Work out the finished part from the listing and answer in its coordinate system (mm). A direction names the side the tool comes from. Give positions to 0.01 mm unless a question says otherwise; leave off trailing zeros. Loops run counter-clockwise (first coordinate to the right, second up) from the corner with the lowest first, then second, coordinate; pieces in that order, holes last. Notation, with made-up numbers: (39.5, 39.25) - (50.5, 39.25) arc R9 ccw to (50.5, 53.25) - close; hole circle Ø7 at (-24, -35.75). An arc over 180 degrees is marked (long way). One line per question, with ' | ' between items. Start each with the question number.
1. Which of the six approach directions +Z, -Z, +X, -X, +Y, -Y give full straight-line access (tool end or side, diameter ignored) to faces 1 (the face through (-69, -3.44, 3)), 2 (the face through (-65.085, -17, 3)), 3 (the face through (-63, -9, 3))?
2. Section B-B (x = -4) is taken. Determine the outline of the cut face in (y, z), plus the area to 3 significant figures.
3. Section C-C (y = 10) is taken. Determine the outline of the cut face in (x, z) (3 decimals), plus the area to 3 significant figures.
4. Each of these flat-tipped pins is pushed along its axis until it touches: pin 1 (2 mm diameter, centred on y = -1.5, z = 4, fed in from -X); pin 2 (1 mm diameter, centred on x = -46.5, z = 3, fed in from +Y). Where does it stop, or does it pass through?
5. Section D-D (z = 3.75) is taken. Give the number of separate pieces and of enclosed holes in the cut face, plus the area to 3 significant figures.
6. Section A-A (y = -10) is taken. Determine the outline of the cut face in (x, z) (3 decimals), plus the area to 3 significant figures.
7. Find the intervals of material crossed by line 1 (Y direction, x = 21, z = 3.75) (3 decimals); line 2 (Y direction, x = -21, z = 3.5) (3 decimals); line 3 (Y direction, x = -2.5, z = 5.25), in increasing order.
8. For a pull along Y with two mould halves and no side action, classify faces 4 (the face through (-45.2, 40.1, 3.3)), 5 (the face through (-22.31, 11.2, 3.25)), 6 (the face through (-50.3, 20, 3)) as released by +Y, released by -Y, zero draft, split by the parting line, or undercut.
from build123d import *

# Parameters (mm, degrees)
MODEL_R             = 1.775
MODEL_W             = 28.5
MODEL_H             = 6.88
BOSS_EXTRUDE1_DEPTH = 6.6


with BuildPart() as part:
    # Model → Boss-Extrude1 (new body)
    with BuildSketch(Plane.XY):
        with BuildLine():
            Line((-40.3, 45), (-50.3, 35))
            Line((-50.3, 35), (-50.3, 5.44))
            ThreePointArc((-50.3, 5.44), (-49.714213562, 4.025786438), (-48.3, 3.44))
            Line((-48.3, 3.44), (-40.7, 3.44))
            Line((-40.7, 3.44), (-40.7, -3.44))
            Line((-40.7, -3.44), (-59.45, -3.44))
            Line((-59.45, -3.44), (-59.45, -14.44))
            Line((-59.45, -14.44), (-57.865, -14.44))
            ThreePointArc((-57.865, -14.44), (-57.511446609, -14.586446609), (-57.365, -14.94))
            Line((-57.365, -14.94), (-57.365, -18.94))
            ThreePointArc((-57.365, -18.94), (-57.511446609, -19.293553391), (-57.865, -19.44))
            Line((-57.865, -19.44), (-59.45, -19.44))
            Line((-59.45, -19.44), (-59.45, -23.94))
            ThreePointArc((-59.45, -23.94), (-59.596446609, -24.293553391), (-59.95, -24.44))
            Line((-59.95, -24.44), (-62.5, -24.44))
            ThreePointArc((-62.5, -24.44), (-62.853553391, -24.293553391), (-63, -23.94))
            Line((-63, -23.94), (-63, -19.44))
            Line((-63, -19.44), (-64.585, -19.44))
            ThreePointArc((-64.585, -19.44), (-64.938553391, -19.293553391), (-65.085, -18.94))
            Line((-65.085, -18.94), (-65.085, -14.94))
            ThreePointArc((-65.085, -14.94), (-64.938553391, -14.586446609), (-64.585, -14.44))
            Line((-64.585, -14.44), (-63, -14.44))
            Line((-63, -14.44), (-63, -3.44))
            Line((-63, -3.44), (-75.7, -3.44))
            Line((-75.7, -3.44), (-75.7, -35))
            Line((-75.7, -35), (-65.7, -45))
            Line((-65.7, -45), (21, -45))
            Line((21, -45), (31, -35))
            Line((31, -35), (31, 35))
            Line((31, 35), (21, 45))
            Line((21, 45), (-40.3, 45))
        make_face()
        with Locations((-21, 30)):
            Circle(MODEL_R, mode=Mode.SUBTRACT)
        with Locations((-21, 10)):
            Circle(MODEL_R, mode=Mode.SUBTRACT)
        with Locations((-21, -10)):
            Circle(MODEL_R, mode=Mode.SUBTRACT)
        with Locations((-21, -30)):
            Circle(MODEL_R, mode=Mode.SUBTRACT)
        with Locations((21, 20)):
            Circle(MODEL_R, mode=Mode.SUBTRACT)
        with Locations((21, -20)):
            Circle(MODEL_R, mode=Mode.SUBTRACT)
        with Locations((-22.524993759, 0)):
            Circle(MODEL_R, mode=Mode.SUBTRACT)
        with Locations((20.525006241, 0)):
            Circle(MODEL_R, mode=Mode.SUBTRACT)
        with Locations((1.500006241, 0)):
            Rectangle(MODEL_W, MODEL_H, mode=Mode.SUBTRACT)
    extrude(amount=BOSS_EXTRUDE1_DEPTH)


solid = part.part
Conclusion:
1) face 1: +Z, -Z, -X, +Y | face 2: +Z, -Z | face 3: +Z, -Z, +Y
2) outline: (-45, 0) - (-3.44, 0) - (-3.44, 6.6) - (-45, 6.6) - close; (3.44, 0) - (45, 0) - (45, 6.6) - (3.44, 6.6) - close | area: 549 mm²
3) outline: (-50.3, 0) - (-22.775, 0) - (-22.775, 6.6) - (-50.3, 6.6) - close; (-19.225, 0) - (31, 0) - (31, 6.6) - (-19.225, 6.6) - close | area: 513 mm²
4) pin 1: x = -40.7 | pin 2: y = 39.3
5) separate pieces: 1 | enclosed holes: 9 | area: 7,740 mm²
6) outline: (-75.7, 0) - (-63, 0) - (-63, 6.6) - (-75.7, 6.6) - close; (-59.45, 0) - (-22.775, 0) - (-22.775, 6.6) - (-59.45, 6.6) - close; (-19.225, 0) - (31, 0) - (31, 6.6) - (-19.225, 6.6) - close | area: 657 mm²
7) line 1: -45 to -21.775, -18.225 to -1.71, 1.71 to 18.225, 21.775 to 45 | line 2: -45 to -31.775, -28.225 to -11.775, -8.225 to -0.908, 0.908 to 8.225, 11.775 to 28.225, 31.775 to 45 | line 3: -45 to -3.44, 3.44 to 45
8) face 4: released by +Y | face 5: undercut | face 6: zero draft
